Can you work these out from the model? Positions are in its coordinate system, mm. A direction names the side the tool comes from. Give positions to 0.01 mm unless a question says otherwise; leave off trailing zeros. Write each loop counter-clockwise with the first axis right and the second up, starting at its lowest first coordinate (ties: lowest second). Pieces come first, ordered by that corner, then holes. Notation, with made-up numbers: (87, -38.5) -> (131, -38.5) arc R25 ccw to (131, -0.5) -> close; hole circle Ø1 at (27, 52.5). An arc over 180 degrees is marked (long way). One line per item, written item: value.
from build123d import *

# Parameters (mm, degrees)
SKETCH004_W   = 110
SKETCH004_H   = 71
SKETCH004_R   = 1.5
SKETCH004_R_2 = 27.5
PAD001_DEPTH  = 3
SKETCH005_W   = 6
SKETCH005_H   = 6
SKETCH005_R   = 1.5
PAD002_DEPTH  = 3


with BuildPart() as coverplane:
    # Sketch004 → Pad001 (new body)
    with BuildSketch(Plane.YZ):
        Rectangle(SKETCH004_W, SKETCH004_H)
        with Locations((25, 25)):
            Circle(SKETCH004_R, mode=Mode.SUBTRACT)
        with Locations((-25, 25)):
            Circle(SKETCH004_R, mode=Mode.SUBTRACT)
        with Locations((25, -25)):
            Circle(SKETCH004_R, mode=Mode.SUBTRACT)
        with Locations((-25, -25)):
            Circle(SKETCH004_R, mode=Mode.SUBTRACT)
        Circle(SKETCH004_R_2, mode=Mode.SUBTRACT)
    extrude(amount=PAD001_DEPTH)

    # Sketch005 → Pad002 (join)
    with BuildSketch(Plane.XY.offset(-35.5)):
        with Locations((-3, 52)):
            Rectangle(SKETCH005_W, SKETCH005_H)
        with Locations((-3, 52)):
            Circle(SKETCH005_R, mode=Mode.SUBTRACT)
        with Locations((-3, -52)):
            Rectangle(SKETCH005_W, SKETCH005_H)
        with Locations((-3, -52)):
            Circle(SKETCH005_R, mode=Mode.SUBTRACT)
    pad002 = extrude(amount=PAD002_DEPTH)

    # Mirrored: Pad002 across XY
    add(pad002.mirror(Plane.XY))


with BuildPart() as part_mirroring:
    # Part__Mirroring: instance of coverplane
    add(coverplane.part.mirror(Plane(origin=(-32.5, 0, 0), x_dir=(0, -1, 0), z_dir=(1, 0, 0))))


solid = part_mirroring.part
1) If we section it at C-C (x = -62): State how many separate pieces and enclosed holes the cut face has, and give its area (3 significant figures).
Answer list:
separate pieces: 8
enclosed holes: 0
area: 36.0 mm^2
2) For faces 5 (the face through (-60.6, -50.6, 32.5)), 6 (the face through (-63.386, 51.425, -34.021)), which set-ups out of +Z, -Z, +X, -X, +Y, -Y let a thin tool reach every point of the face, with its end or its side?
Answer list:
face 5: +X, +Y, -Y
face 6: +Z, -Z
3) We'd pull the mould along Y, two halves only. Please class faces 1 (the face through (-65.4, 13, -35.5)), 2 (the face through (-62, 49, -34)), 3 (the face through (-66, 55, 0)), 4 (the face through (-66.48, -26.11, 26.01)): released by +Y, released by -Y, zero draft, split by the parting line, or undercut.
Answer list:
face 1: zero draft
face 2: undercut
face 3: released by +Y
face 4: undercut
4) I need wall thicknesses on L1, parallel to Y at x = -62, z = -34.1; L2, parallel to X at y = 30, z = -21.5; L3, parallel to Y at x = -66.25, z = -24.5. Which ranges of each line are inside material? Lowest first, please.
Answer list:
L1: y = -55 to -53.5, -50.5 to -49, 49 to 50.5, 53.5 to 55
L2: x = -68 to -65
L3: y = -55 to -26.41, -23.59 to -12.49, 12.49 to 23.59, 26.41 to 55
5) Will these pins go through, and if not, where does the flat tip stop? pin 1 (1.8 mm diameter, centred on x = -62.5, y = 52.5, fed in from -Z); pin 2 (3.5 mm diameter, centred on y = -25, z = -25, fed in from +X).
Answer list:
pin 1: stops at z = -35.5
pin 2: stops at x = -65
6) If we section it at A-A (z = 0): Write out the boundary of the cut face in (x, y).
Answer list:
outline: (-68, -55) -> (-65, -55) -> (-65, -27.5) -> (-68, -27.5) -> close; (-68, 27.5) -> (-65, 27.5) -> (-65, 55) -> (-68, 55) -> close
7) If we section it at D-D (y = -15): Write out the boundary of the cut face in (x, z), and give its area (3 significant figures).
Answer list:
outline: (-68, -35.5) -> (-65, -35.5) -> (-65, -23.05) -> (-68, -23.05) -> close; (-68, 23.05) -> (-65, 23.05) -> (-65, 35.5) -> (-68, 35.5) -> close
area: 74.7 mm^2
8) If we section it at B-B (y = 52): Write out the boundary of the cut face in (x, z).
Answer list:
outline: (-68, -35.5) -> (-63.5, -35.5) -> (-63.5, -32.5) -> (-65, -32.5) -> (-65, 32.5) -> (-63.5, 32.5) -> (-63.5, 35.5) -> (-68, 35.5) -> close; (-60.5, -35.5) -> (-59, -35.5) -> (-59, -32.5) -> (-60.5, -32.5) -> close; (-60.5, 32.5) -> (-59, 32.5) -> (-59, 35.5) -> (-60.5, 35.5) -> close
